```python
from build123d import *

# Parameters (mm, degrees)
BOSS_EXTRUDE1_DEPTH = 5
CUT_EXTRUDE1_DEPTH  = 5
SKETCH4_R           = 2
CUT_EXTRUDE2_DEPTH  = 5


with BuildPart() as part:
    # Sketch1 → Boss-Extrude1 (new body)
    with BuildSketch(Plane.XY):
        Polygon((10, -22.5), (47.5, -22.5), (47.5, 22.5), (-47.5, 22.5), (-47.5, -22.5), (-10, -22.5), (-10, -27.4), (10, -27.4), align=None)
    extrude(amount=BOSS_EXTRUDE1_DEPTH)

    # Sketch3 → Cut-Extrude1 (cut)
    with BuildSketch(Plane.XY.offset(5)):
        Polygon((-33.1, -19.5), (-33.1, -22.5), (-37.5, -22.5), (-37.5, -19.5), (-39, -19.5), (-39, -16.1), (-37.5, -16.1), (-37.5, -9.1), (-33.1, -9.1), (-33.1, -16.1), (-31.6, -16.1), (-31.6, -19.5), align=None)
        Polygon((37.5, -22.5), (37.5, -19.5), (39, -19.5), (39, -16.1), (37.5, -16.1), (37.5, -9.1), (33.1, -9.1), (33.1, -16.1), (31.6, -16.1), (31.6, -19.5), (33.1, -19.5), (33.1, -22.5), align=None)
        Polygon((33.1, 19.5), (33.1, 22.5), (37.5, 22.5), (37.5, 19.5), (39, 19.5), (39, 16.1), (37.5, 16.1), (37.5, 9.1), (33.1, 9.1), (33.1, 16.1), (31.6, 16.1), (31.6, 19.5), align=None)
        Polygon((-32.5, 19.5), (-32.5, 22.5), (-28.1, 22.5), (-28.1, 19.5), (-26.6, 19.5), (-26.6, 16.1), (-28.1, 16.1), (-28.1, 9.1), (-32.5, 9.1), (-32.5, 16.1), (-34, 16.1), (-34, 19.5), align=None)
    extrude(amount=-CUT_EXTRUDE1_DEPTH, mode=Mode.SUBTRACT)

    # Sketch4 → Cut-Extrude2 (cut)
    with BuildSketch(Plane.XY.offset(5)):
        with Locations((10, -2.2)):
            Circle(SKETCH4_R)
    extrude(amount=-CUT_EXTRUDE2_DEPTH, mode=Mode.SUBTRACT)


solid = part.part
```
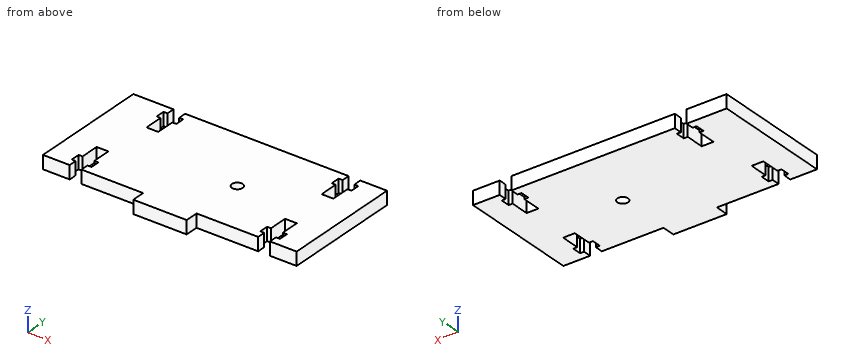
CAD build for the part. Positions are in the model's coordinates, mm. Round coordinates to 2 decimals unless told otherwise and drop trailing zeros. Order: outer loops, then holes, each group sorted by start corner. A loop starts at its lowest first (then second) coordinate and runs counter-clockwise, first axis right, second up. Notation, with made-up numbers: (45, -34.5) - (89, -34.5) arc R21 ccw to (89, -4.5) - close; hole circle Ø5 at (72, -17.5). An arc over 180 degrees is marked (long way). Answer in a Markdown table with one row per item. Add a question column.
(1) Band-saw the part on B-B on y = -2.2. List the corners of the cut face in (x, z).
(2) Probe L1, parallel to X at y = -19, z = 1.1; L2, parallel to X at y = -21, z = 0.95; L3, parallel to X at y = -24, z = 0.7. List the from-to ranges inside material, lowest first. Write a range as [from, to].
(3) Band-saw the part on A-A on y = 17. List the corners of the cut face in (x, z), and give its area (3 significant figures).
(4) Band-saw the part on C-C on x = 30. List the corners of the cut face in (y, z), and give its area (3 significant figures).
(5) Drop a flat-ended pin along its axis: pin 1 Ø2 at (x, z) = (29, 4.5) entering from -Y. Give the stop position or say it passes through.
(6) Band-saw the part on D-D on y = 10.5. List the corners of the cut face in (x, z).
Data:
| question | item | result |
|---|---|---|
| 1 | outline | (-47.5, 0) - (8, 0) - (8, 5) - (-47.5, 5) - close; (12, 0) - (47.5, 0) - (47.5, 5) - (12, 5) - close |
| 2 | L1 | x = [-47.5, -39], [-31.6, 31.6], [39, 47.5] |
| 2 | L2 | x = [-47.5, -37.5], [-33.1, 33.1], [37.5, 47.5] |
| 2 | L3 | x = [-10, 10] |
| 3 | outline | (-47.5, 0) - (-34, 0) - (-34, 5) - (-47.5, 5) - close; (-26.6, 0) - (31.6, 0) - (31.6, 5) - (-26.6, 5) - close; (39, 0) - (47.5, 0) - (47.5, 5) - (39, 5) - close |
| 3 | area | 401 mm^2 |
| 4 | outline | (-22.5, 0) - (22.5, 0) - (22.5, 5) - (-22.5, 5) - close |
| 4 | area | 225 mm^2 |
| 5 | pin 1 | stops at y = -22.5 |
| 6 | outline | (-47.5, 0) - (-32.5, 0) - (-32.5, 5) - (-47.5, 5) - close; (-28.1, 0) - (33.1, 0) - (33.1, 5) - (-28.1, 5) - close; (37.5, 0) - (47.5, 0) - (47.5, 5) - (37.5, 5) - close |
